The drawing under review shows one solid part. Ordinate dimensions are in mm from its lowest x, y, z. A direction names the side the tool comes from. Round coordinates to 2 decimals unless told otherwise and drop trailing zeros. Order: outer loops, then holes, each group sorted by start corner. A loop starts at its lowest first (then second) coordinate and runs counter-clockwise, first axis right, second up. Notation, with made-up numbers: M 43.25,18 L 79.25,18 A14 ccw 79.25,29 Z; hole C -10.75,33.25 d4. An arc over 180 degrees is marked long. Answer as a JSON object with one key per item and string values. Group by question number.
1. Add section B-B on y = 9.25. State the section outline as (x, z) points.
2. Mouldability with a two-part tool opening along X and no side actions: class the marked faces 3, 4 and 5 as released by +X, released by -X, zero draft, split by the parting line, or undercut.
3. Machinability: for the marked faces 1 and 2, which of the approach directions +Z, -Z, +X, -X, +Y, -Y give a long, thin tool a straight path to every point of the face, cutting with its end or side? Answer none if there is none.
4. Add section C-C on x = 24. State the section outline as (y, z) points, and give its area (3 significant figures).
5. Clearance check with a flat-ended pin moving along its axis: P1, Ø3, axis at x = 22.5, y = 5, coming from the -Z side. State where the tip first meets the part, or that it passes through.
6. To check wall thickness, follow probe 1 along X at (y, z) = (6.25, 13.5); probe 2 along Z at (x, y) = (50, 3.75); probe 3 along X at (y, z) = (4.5, 1) (3 decimals). State the ranges of each line that lie inside material, in increasing order. Write a range as [from, to].
7. Add section A-A on z = 10.5. State the section outline as (x, y) points, and give its area (3 significant figures).
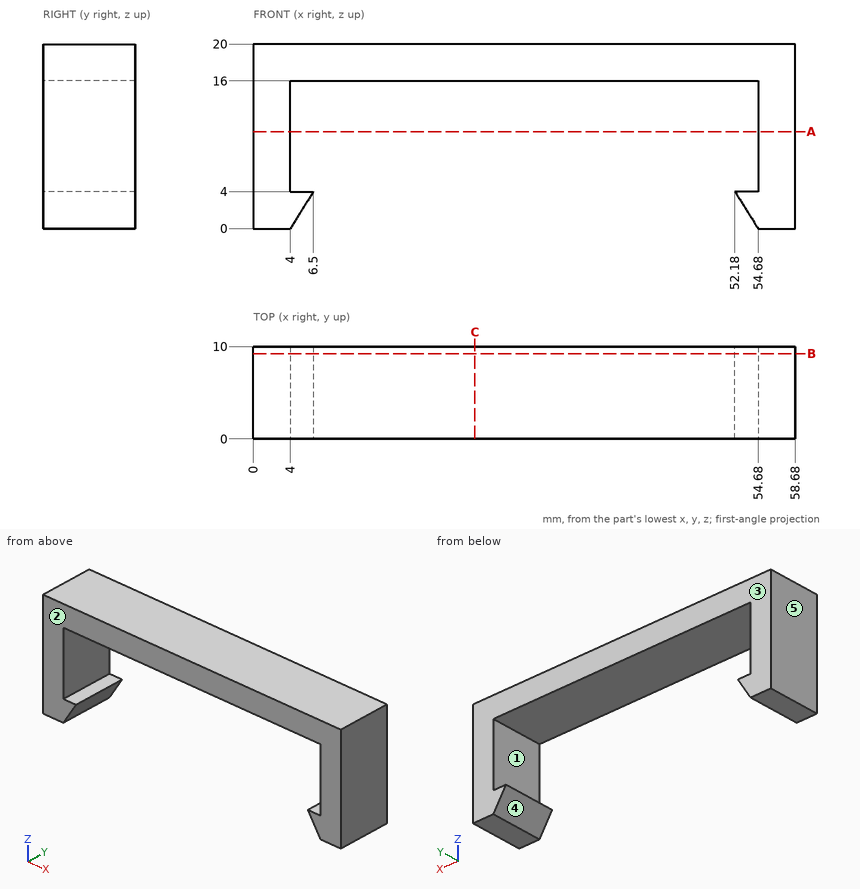
Recorded:
{
 "1": {"outline": "M 0,0 L 4,0 L 6.5,4 L 4,4 L 4,16 L 54.68,16 L 54.68,4 L 52.18,4 L 54.68,0 L 58.68,0 L 58.68,20 L 0,20 Z"},
 "2": {"face 3": "zero draft", "face 4": "undercut", "face 5": "released by -X"},
 "3": {"face 1": "+Y, -Y", "face 2": "+Z, -Z, +X, -X, -Y"},
 "4": {"outline": "M 0,16 L 10,16 L 10,20 L 0,20 Z", "area": "40.0 mm²"},
 "5": {"P1": "stops at z = 16"},
 "6": {"probe 1": "x = [0, 4], [54.68, 58.68]", "probe 2": "z = [16, 20]", "probe 3": "x = [0, 4.625], [54.055, 58.68]"},
 "7": {"outline": "M 0,0 L 4,0 L 4,10 L 0,10 Z; M 54.68,0 L 58.68,0 L 58.68,10 L 54.68,10 Z", "area": "80.0 mm²"}
}
